Model file for the job. Use its own axes, mm. Coordinates: 2 decimals unless noted, no trailing zeros. Loops run counter-clockwise (first coordinate to the right, second up) from the corner with the lowest first, then second, coordinate; pieces in that order, holes last. Notation, with made-up numbers: M 11,-10 L 39,-10 A14 cw 39,5 Z; hole C 58,16 d6. An arc over 180 degrees is marked long. One line per question, with ' | ' between items. Start each with the question number.
```python
from build123d import *

# Parameters (mm, degrees)
SKETCH1_W           = 190.5
SKETCH1_H           = 304.8
BOSS_EXTRUDE1_DEPTH = 2.778125
SKETCH2_W           = 190.5
SKETCH2_H           = 17.78
CUT_EXTRUDE1_DEPTH  = 3.778125
SKETCH3_W           = 17.78
SKETCH3_H           = 269.24
CUT_EXTRUDE2_DEPTH  = 3.778125
CUT_EXTRUDE3_DEPTH  = 3.778125
FILLET1_R           = 2.54


with BuildPart() as part:
    # Sketch1 → Boss-Extrude1 (new body)
    with BuildSketch(Plane(origin=(0, 0, 0), x_dir=(1, 0, 0), z_dir=(0, 1, 0))):
        with Locations((95.25, 152.4)):
            Rectangle(SKETCH1_W, SKETCH1_H)
    extrude(amount=BOSS_EXTRUDE1_DEPTH)

    # Sketch2 → Cut-Extrude1 (cut, through all)
    with BuildSketch(Plane(origin=(0, 2.778125, 0), x_dir=(1, 0, 0), z_dir=(0, 1, 0))):
        with Locations((95.25, 8.89)):
            Rectangle(SKETCH2_W, SKETCH2_H)
        with Locations((95.25, 295.91)):
            Rectangle(SKETCH2_W, SKETCH2_H)
    extrude(amount=-CUT_EXTRUDE1_DEPTH, mode=Mode.SUBTRACT)

    # Sketch3 → Cut-Extrude2 (cut, through all)
    with BuildSketch(Plane(origin=(0, 2.778125, 0), x_dir=(1, 0, 0), z_dir=(0, 1, 0))):
        with Locations((8.89, 152.4)):
            Rectangle(SKETCH3_W, SKETCH3_H)
    extrude(amount=-CUT_EXTRUDE2_DEPTH, mode=Mode.SUBTRACT)

    # Sketch4 → Cut-Extrude3 (cut, through all)
    with BuildSketch(Plane(origin=(0, 2.778125, 0), x_dir=(1, 0, 0), z_dir=(0, 1, 0))):
        Polygon((17.78, 287.02), (76.454, 287.02), (76.454, 269.875), (34.925, 269.875), (34.925, 228.346), (17.78, 228.346), align=None)
        Polygon((17.78, 17.78), (76.454, 17.78), (76.454, 34.925), (34.925, 34.925), (34.925, 76.454), (17.78, 76.454), align=None)
    extrude(amount=-CUT_EXTRUDE3_DEPTH, mode=Mode.SUBTRACT)

    # Fillet1
    fillet1_edges = [part.edges().sort_by_distance(p)[0] for p in [
        (190.5, 1.3890625, -17.78),
        (190.5, 1.3890625, -287.02),
        (17.78, 1.3890625, -228.346),
        (76.454, 1.3890625, -287.02),
        (76.454, 1.3890625, -269.875),
        (34.925, 1.3890625, -269.875),
        (34.925, 1.3890625, -228.346),
        (17.78, 1.3890625, -76.454),
        (34.925, 1.3890625, -76.454),
        (34.925, 1.3890625, -34.925),
        (76.454, 1.3890625, -34.925),
        (76.454, 1.3890625, -17.78),
    ]]
    fillet(fillet1_edges, radius=FILLET1_R)


solid = part.part
```
(1) Band-saw the part on C-C on z = -68. Write the cut outline in (x, y) (3 decimals).
(2) Band-saw the part on B-B on x = 50. Write the cut outline in (y, z) (3 decimals).
(3) Drill centre lines: line 1 (X direction, y = 1.35, z = -233) (3 decimals); line 2 (Z direction, x = 64, y = 1.1) (3 decimals); line 3 (X direction, y = 0.3, z = -269). Where is each one in solid material? Low to high. Write a range as [from, to].
(4) Pin check, flat tips, straight feed: P1, Ø1, axis at x = 45.5, y = 0.5, coming from the -Z side (3 decimals); P2, Ø1.4, axis at x = 26.5, y = 0.5, coming from the -Z side; P3, Ø1.4, axis at y = 1, z = -62, coming from the -X side (3 decimals). Stop position of each tip, or through.
(5) Band-saw the part on A-A on y = 0.55. Write the cut outline in (x, z) (3 decimals).
Computed values:
1) outline: M 34.925,0 L 190.5,0 L 190.5,2.778 L 34.925,2.778 Z
2) outline: M 0,-269.875 L 2.778,-269.875 L 2.778,-34.925 L 0,-34.925 Z
3) line 1: [34.925, 190.5] | line 2: [-269.875, -34.925] | line 3: [35.55, 190.5]
4) P1: z = -269.875 | P2: z = -228.35 | P3: x = 34.925
5) outline: M 17.78,-225.806 A2.54 ccw 20.32,-228.346 L 32.385,-228.346 A2.54 cw 34.925,-230.886 L 34.925,-267.335 A2.54 ccw 37.465,-269.875 L 73.914,-269.875 A2.54 cw 76.454,-272.415 L 76.454,-284.48 A2.54 ccw 78.994,-287.02 L 187.96,-287.02 A2.54 ccw 190.5,-284.48 L 190.5,-20.32 A2.54 ccw 187.96,-17.78 L 78.994,-17.78 A2.54 ccw 76.454,-20.32 L 76.454,-32.385 A2.54 cw 73.914,-34.925 L 37.465,-34.925 A2.54 ccw 34.925,-37.465 L 34.925,-73.914 A2.54 cw 32.385,-76.454 L 20.32,-76.454 A2.54 ccw 17.78,-78.994 Z
